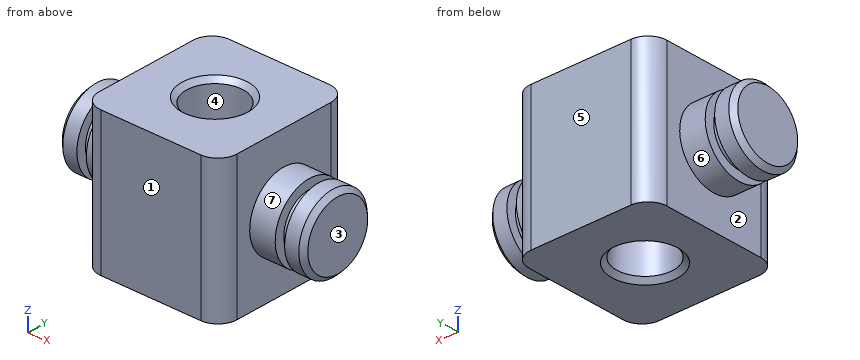
from build123d import *

# Parameters (mm, degrees)
SKETCH1_R                = 3
BOSS_EXTRUDE1_DEPTH      = 15
SKETCH2_R                = 4
BOSS_EXTRUDE2_DEPTH      = 2.7
SKETCH3_R                = 3
BOSS_EXTRUDE3_DEPTH      = 1
SKETCH4_R                = 4
BOSS_EXTRUDE4_DEPTH      = 2
CHAMFER1_SIZE            = 0.5
CHAMFER1_OF_MIRROR1_SIZE = 0.5
CHAMFER2_SIZE            = 0.5


with BuildPart() as part:
    # Sketch1 → Boss-Extrude1 (new body)
    with BuildSketch(Plane.XY):
        with BuildLine():
            Line((-5.3, -7.5), (5.3, -7.5))
            ThreePointArc((5.3, -7.5), (6.714213562, -6.914213562), (7.3, -5.5))
            Line((7.3, -5.5), (7.3, 5.5))
            ThreePointArc((7.3, 5.5), (6.714213562, 6.914213562), (5.3, 7.5))
            Line((5.3, 7.5), (-5.3, 7.5))
            ThreePointArc((-5.3, 7.5), (-6.714213562, 6.914213562), (-7.3, 5.5))
            Line((-7.3, 5.5), (-7.3, -5.5))
            ThreePointArc((-7.3, -5.5), (-6.714213562, -6.914213562), (-5.3, -7.5))
        make_face()
        Circle(SKETCH1_R, mode=Mode.SUBTRACT)
    extrude(amount=BOSS_EXTRUDE1_DEPTH)

    # Sketch2 → Boss-Extrude2 (add)
    with BuildSketch(Plane.ZY.offset(7.3)):
        with Locations(Location((7.5, 0, 0), (0, 0, 180))):
            Circle(SKETCH2_R)
    boss_extrude2 = extrude(amount=BOSS_EXTRUDE2_DEPTH)

    # Sketch3 → Boss-Extrude3 (add)
    with BuildSketch(Plane.ZY.offset(10)):
        with Locations((7.5, 0)):
            Circle(SKETCH3_R)
    boss_extrude3 = extrude(amount=BOSS_EXTRUDE3_DEPTH)

    # Sketch4 → Boss-Extrude4 (add)
    with BuildSketch(Plane.ZY.offset(11)):
        with Locations(Location((7.5, 0, 0), (0, 0, 180))):
            Circle(SKETCH4_R)
    boss_extrude4 = extrude(amount=BOSS_EXTRUDE4_DEPTH)

    # Chamfer1
    chamfer1_edges = [part.edges().sort_by_distance(p)[0] for p in [
        (-13, 0, 11.5),
    ]]
    chamfer(chamfer1_edges, length=CHAMFER1_SIZE)

    # Mirror1: Boss-Extrude2, Boss-Extrude3, Boss-Extrude4 across plane
    add(boss_extrude2.mirror(Plane(origin=(0, 0, 0), x_dir=(0, 0, 1), z_dir=(1, 0, 0))))
    add(boss_extrude3.mirror(Plane(origin=(0, 0, 0), x_dir=(0, 0, 1), z_dir=(1, 0, 0))))
    add(boss_extrude4.mirror(Plane(origin=(0, 0, 0), x_dir=(0, 0, 1), z_dir=(1, 0, 0))))

    # Chamfer1 of Mirror1
    chamfer1_of_mirror1_edges = [part.edges().sort_by_distance(p)[0] for p in [
        (13, 0, 11.5),
    ]]
    chamfer(chamfer1_of_mirror1_edges, length=CHAMFER1_OF_MIRROR1_SIZE)

    # Chamfer2
    chamfer2_edges = [part.edges().sort_by_distance(p)[0] for p in [
        (-3, 0, 0),
        (-3, 0, 15),
    ]]
    chamfer(chamfer2_edges, length=CHAMFER2_SIZE)


solid = part.part
Source: CAD feature listing. Evaluate the final solid. Frame: model axes, mm. Face numbers are marked on the shaded views. A direction names the side the tool comes from. Give positions to 0.01 mm unless a question says otherwise; leave off trailing zeros. Order: outer loops, then holes, each group sorted by start corner. A loop starts at its lowest first (then second) coordinate and runs counter-clockwise, first axis right, second up. Notation, with made-up numbers: (-26.5, -1.75) -> (-4.5, -1.75) arc R17 ccw to (-4.5, 13.25) -> close; hole circle Ø10 at (53.25, -2). An arc over 180 degrees is marked (long way). Use a Markdown table: item, result.
1) Ray query, line 1 along Y through (x, z) = (0, 11); line 2 along X through (y, z) = (-3.75, 12); line 3 along X through (y, z) = (0.5, 13). Return the intervals inside material, ascending. Write a range as [from, to].
Answer list:
| item | result |
|---|---|
| line 1 | [-7.5, -3], [3, 7.5] |
| line 2 | [-7.3, 7.3] |
| line 3 | [-7.3, -2.96], [2.96, 7.3] |
2) Mould query, pull axis X, two halves, no side actions, for the marked faces 1, 2, 3 and 4. Classes: +X half, -X half, draft (parallel to the pull), parting line (faces both ways), or undercut.
Answer list:
| item | result |
|---|---|
| face 1 | draft |
| face 2 | -X half |
| face 3 | +X half |
| face 4 | undercut |
3) Section query A-A, the plane z = 14. Return the cut outline in (x, y).
Answer list:
| item | result |
|---|---|
| outline | (-7.3, -5.5) arc R2 ccw to (-5.3, -7.5) -> (5.3, -7.5) arc R2 ccw to (7.3, -5.5) -> (7.3, 5.5) arc R2 ccw to (5.3, 7.5) -> (-5.3, 7.5) arc R2 ccw to (-7.3, 5.5) -> close; hole circle Ø6 at (0, 0) |
4) Section query B-B, the plane x = 0. Return the cut outline in (y, z).
Answer list:
| item | result |
|---|---|
| outline | (-7.5, 0) -> (-3.5, 0) -> (-3, 0.5) -> (-3, 14.5) -> (-3.5, 15) -> (-7.5, 15) -> close; (3, 0.5) -> (3.5, 0) -> (7.5, 0) -> (7.5, 15) -> (3.5, 15) -> (3, 14.5) -> close |
5) Section query D-D, the plane x = 10.5. Return the cut outline in (y, z), then the cut area to 3 significant figures.
Answer list:
| item | result |
|---|---|
| outline | circle Ø6 at (0, 7.5) |
| area | 28.3 mm² |
6) Contact query for flat-ended pins moving along their axis: P1, Ø2, axis at y = -5.5, z = 7, coming from the -X side; P2, Ø1.5, axis at x = -8.5, z = 6, coming from the -Y side. Output: stop coordinate, or through.
Answer list:
| item | result |
|---|---|
| P1 | x = -7.3 |
| P2 | y = -3.93 |
7) Reachability of the marked faces 5, 6 and 7 from +Z, -Z, +X, -X, +Y, -Y: full face, straight path, thin tool, end or side. Return the list, or none.
Answer list:
| item | result |
|---|---|
| face 5 | +Z, -Z, +X, -X, +Y |
| face 6 | -X |
| face 7 | +X |
8) Section query C-C, the plane y = 4.5. Return the cut outline in (x, z), then the cut area to 3 significant figures.
Answer list:
| item | result |
|---|---|
| outline | (-7.3, 0) -> (7.3, 0) -> (7.3, 15) -> (-7.3, 15) -> close |
| area | 219 mm² |
